Read the model definition and answer for the solid it produces. Units are mm, in the model's axes. Give positions to 0.01 mm unless a question says otherwise; leave off trailing zeros. Loops run counter-clockwise (first coordinate to the right, second up) from the corner with the lowest first, then second, coordinate; pieces in that order, holes last. Notation, with made-up numbers: (31.25, 59) - (80.25, 59) arc R12 cw to (80.25, 67) - close; hole circle Ø2 at (-20.75, 63.5). An arc over 180 degrees is marked (long way). Write each question's results on one line, items separated by ' | '. Start each with the question number.
Q1. Find the intervals of material crossed by line 1 (Z direction, x = -19.05, y = -8); line 2 (Z direction, x = -19.05, y = -4.5); line 3 (Z direction, x = -23.5, y = -10.5), in increasing order. Write a range as from..to.
Q2. The part is cut by section C-C, the plane y = -8.75. Write down the section's boundary in (x, z).
Q3. Given pin 1 (8.5 mm diameter, centred on x = -19.05, z = 15.24, fed in from +Y), flat-ended and moving along its own axis, determine where the tip first touches the part or whether it passes through.
Q4. The part is cut by section D-D, the plane x = -10.5. Write down the section's boundary in (y, z) (3 decimals), plus the area to 3 significant figures.
Q5. The part is cut by section B-B, the plane x = -19.05. Write down the section's boundary in (y, z) (3 decimals).
Q6. Determine the mould class of faces 1 (the flat face through (-19, -19.05, 26)), 2 (the flat face through (-19, -9, 50.8)), 3 (the flat face through (-19, 0, 26)), 4 (the cylindrical face through (-19.317, -12.553, 39.054)) for opening direction Y: +Y half, -Y half, draft (parallel to the pull), parting line (faces both ways), or undercut.
Q7. The part is cut by section A-A, the plane z = 15.24. Write down the section's boundary in (x, y), plus the area to 3 significant figures.
```python
from build123d import *

# Parameters (mm, degrees)
F0_W     = 38.1
F0_H     = 50.8
F1_DEPTH = 19.05
F3_D     = 6.35
F4_D     = 10.71626


with BuildPart() as f1:
    # F0 (on Front) → F1 (new body)
    with BuildSketch(Plane.XZ):
        with Locations((-19.05, 25.4)):
            Rectangle(F0_W, F0_H)
    extrude(amount=F1_DEPTH)

    # F3 (through all)
    with Locations(Plane.YZ):
        with Locations((-9.525, 38.1)):
            Hole(F3_D / 2)

    # F4 (through all)
    with Locations(Plane(origin=(0, 0, 0), x_dir=(1, 0, 0), z_dir=(0, 1, 0))):
        with Locations((-19.05, -15.24)):
            Hole(F4_D / 2)


solid = f1.part
```
Check sheet entries:
1) line 1: z = 0..9.88, 20.6..35.32, 40.88..50.8 | line 2: z = 0..9.88, 20.6..50.8 | line 3: z = 0..12.26, 18.22..35.08, 41.12..50.8
2) outline: (-38.1, 0) - (0, 0) - (0, 35.02) - (-38.1, 35.02) - close; (-38.1, 41.18) - (0, 41.18) - (0, 50.8) - (-38.1, 50.8) - close; hole circle Ø10.72 at (-19.05, 15.24)
3) pin 1: passes through
4) outline: (-19.05, 0) - (0, 0) - (0, 50.8) - (-19.05, 50.8) - close; hole circle Ø6.35 at (-9.525, 38.1) | area: 936 mm^2
5) outline: (-19.05, 0) - (0, 0) - (0, 9.882) - (-19.05, 9.882) - close; (-19.05, 20.598) - (0, 20.598) - (0, 50.8) - (-19.05, 50.8) - close; hole circle Ø6.35 at (-9.525, 38.1)
6) face 1: -Y half | face 2: draft | face 3: +Y half | face 4: undercut
7) outline: (-38.1, -19.05) - (-24.41, -19.05) - (-24.41, 0) - (-38.1, 0) - close; (-13.69, -19.05) - (0, -19.05) - (0, 0) - (-13.69, 0) - close | area: 522 mm^2
